from build123d import *

# Parameters (mm, degrees)
SKETCH1_R           = 6.35
BOSS_EXTRUDE1_DEPTH = 36.195
CHAMFER1_SIZE       = 4.92
CHAMFER2_SIZE       = 1.016
FILLET1_R           = 1.016
SKETCH2_R           = 10.4775
CUT_EXTRUDE1_DEPTH  = 3.175
CUT_EXTRUDE2_START  = -3.175
SKETCH3_R           = 10.4775
CUT_EXTRUDE2_DEPTH  = 3.175
SKETCH4_R           = 2.1082
CUT_EXTRUDE3_DEPTH  = 29.337
CHAMFER3_SIZE       = 1.016


with BuildPart() as part:
    # Sketch1 → Boss-Extrude1 (new body)
    with BuildSketch(Plane(origin=(0, 0, 0), x_dir=(1, 0, 0), z_dir=(0, 1, 0))):
        Polygon((-21, -13.97), (-6.985, -13.97), (-6.985, -13.208), (6.985, -13.208), (6.985, -13.97), (21, -13.97), (21, -5.194), (19.939, -5.194), (19.939, 9.011817488), (11.049, 9.011817488), (11.049, 13.97), (-11.049, 13.97), (-11.049, 9.011817488), (-19.939, 9.011817488), (-19.939, -5.194), (-21, -5.194), align=None)
        with Locations(Location((0, 1.27, 0), (0, 0, 270))):
            Circle(SKETCH1_R, mode=Mode.SUBTRACT)
    extrude(amount=BOSS_EXTRUDE1_DEPTH)

    # Chamfer1
    chamfer1_edges = [part.edges().sort_by_distance(p)[0] for p in [
        (-11.049, 18.0975, -13.97),
        (11.049, 18.0975, -13.97),
    ]]
    chamfer(chamfer1_edges, length=CHAMFER1_SIZE)

    # Chamfer2
    # the kernel refuses this chamfer: 1.016 mm, written as the material it takes off along each edge
    with BuildSketch(Plane(origin=(6.985, -2.612829916, 13.97), x_dir=(0.9996219169112968, 0, 0.027495876610587285), z_dir=(0, 1, 0))) as chamfer2_piece_1_section:
        Polygon((CHAMFER2_SIZE * 0.999621916911, CHAMFER2_SIZE * 0.0274958766106), (-CHAMFER2_SIZE * 0.0274958766106, CHAMFER2_SIZE * 0.999621916911), (0, 0), align=None)
    chamfer2_piece_1 = extrude(amount=41.420659832, mode=Mode.PRIVATE)
    chamfer2_piece_1 = split(chamfer2_piece_1, bisect_by=Plane(origin=(7.342590456, 18.0975, 13.208), z_dir=(0, 0, 1)), keep=Keep.TOP, mode=Mode.PRIVATE)
    add(chamfer2_piece_1, mode=Mode.SUBTRACT)
    with BuildSketch(Plane(origin=(-6.985, -2.612829916, 13.97), x_dir=(0.027495876610586455, 0, -0.9996219169112968), z_dir=(0, 1, 0))) as chamfer2_piece_2_section:
        Polygon((CHAMFER2_SIZE * 0.999621916911, CHAMFER2_SIZE * 0.0274958766106), (-CHAMFER2_SIZE * 0.0274958766106, CHAMFER2_SIZE * 0.999621916911), (0, 0), align=None)
    chamfer2_piece_2 = extrude(amount=41.420659832, mode=Mode.PRIVATE)
    chamfer2_piece_2 = split(chamfer2_piece_2, bisect_by=Plane(origin=(-7.342590456, 18.0975, 13.208), z_dir=(0, 0, 1)), keep=Keep.TOP, mode=Mode.PRIVATE)
    add(chamfer2_piece_2, mode=Mode.SUBTRACT)
    with BuildSketch(Plane(origin=(-21, -2.612829916, 5.194), x_dir=(0.9996219169112968, 0, -0.02749587661058551), z_dir=(0, 1, 0))) as chamfer2_piece_3:
        Polygon((CHAMFER2_SIZE * 0.999621916911, -CHAMFER2_SIZE * 0.0274958766106), (-CHAMFER2_SIZE * 0.0274958766106, -CHAMFER2_SIZE * 0.999621916911), (0, 0), align=None)
    extrude(amount=41.420659832, mode=Mode.SUBTRACT)
    with BuildSketch(Plane(origin=(21, -2.612829916, 5.194), x_dir=(-0.9996219169112968, 0, -0.027495876610584665), z_dir=(0, 1, 0))) as chamfer2_piece_4:
        Polygon((CHAMFER2_SIZE * 0.999621916911, CHAMFER2_SIZE * 0.0274958766106), (-CHAMFER2_SIZE * 0.0274958766106, CHAMFER2_SIZE * 0.999621916911), (0, 0), align=None)
    extrude(amount=41.420659832, mode=Mode.SUBTRACT)

    # Fillet1
    fillet1_edges = [part.edges().sort_by_distance(p)[0] for p in [
        (-19.939, 18.0975, -9.011817488),
        (19.939, 18.0975, -9.011817488),
        (-6.129, 18.0975, -13.97),
        (6.129, 18.0975, -13.97),
    ]]
    fillet(fillet1_edges, radius=FILLET1_R)

    # Sketch2 → Cut-Extrude1 (cut)
    with BuildSketch(Plane(origin=(0, 36.195, 0), x_dir=(1, 0, 0), z_dir=(0, 1, 0))):
        with Locations(Location((0, 1.27, 0), (0, 0, 270))):
            Circle(SKETCH2_R)
    extrude(amount=-CUT_EXTRUDE1_DEPTH, mode=Mode.SUBTRACT)

    # Sketch3 → Cut-Extrude2 (cut)
    with BuildSketch(Plane.XZ.offset(CUT_EXTRUDE2_START)):
        with Locations(Location((0, -1.27, 0), (0, 0, 90))):
            Circle(SKETCH3_R)
    extrude(amount=CUT_EXTRUDE2_DEPTH, mode=Mode.SUBTRACT)

    # Sketch4 → Cut-Extrude3 (cut)
    with BuildSketch(Plane(origin=(0, 0, -9.011817488), x_dir=(-1, 0, 0), z_dir=(0, 0, -1))):
        with Locations((-15.875, 4.7625)):
            Circle(SKETCH4_R)
        with Locations((-15.875, 31.4325)):
            Circle(SKETCH4_R)
        with Locations((15.875, 31.4325)):
            Circle(SKETCH4_R)
        with Locations((15.875, 4.7625)):
            Circle(SKETCH4_R)
    extrude(amount=-CUT_EXTRUDE3_DEPTH, mode=Mode.SUBTRACT)

    # Chamfer3
    # the kernel refuses this chamfer: 1.016 mm, written as the material it takes off along each edge
    with BuildSketch(Plane(origin=(-15.875, 4.7625, -9.011817488), x_dir=(-1, 0, 0), z_dir=(0, -1, 0))) as chamfer3_piece_1:
        Polygon((2.1082 + CHAMFER3_SIZE, 0), (2.1082, -CHAMFER3_SIZE), (2.1082, 0), align=None)
    revolve(axis=Axis((-15.875, 4.7625, -9.011817488), (0, 0, -1)), mode=Mode.SUBTRACT)
    with BuildSketch(Plane(origin=(-15.875, 31.4325, -9.011817488), x_dir=(-1, 0, 0), z_dir=(0, -1, 0))) as chamfer3_piece_2:
        Polygon((2.1082 + CHAMFER3_SIZE, 0), (2.1082, -CHAMFER3_SIZE), (2.1082, 0), align=None)
    revolve(axis=Axis((-15.875, 31.4325, -9.011817488), (0, 0, -1)), mode=Mode.SUBTRACT)
    with BuildSketch(Plane(origin=(15.875, 31.4325, -9.011817488), x_dir=(-1, 0, 0), z_dir=(0, -1, 0))) as chamfer3_piece_3:
        Polygon((2.1082 + CHAMFER3_SIZE, 0), (2.1082, -CHAMFER3_SIZE), (2.1082, 0), align=None)
    revolve(axis=Axis((15.875, 31.4325, -9.011817488), (0, 0, -1)), mode=Mode.SUBTRACT)
    with BuildSketch(Plane(origin=(15.875, 4.7625, -9.011817488), x_dir=(-1, 0, 0), z_dir=(0, -1, 0))) as chamfer3_piece_4:
        Polygon((2.1082 + CHAMFER3_SIZE, 0), (2.1082, -CHAMFER3_SIZE), (2.1082, 0), align=None)
    revolve(axis=Axis((15.875, 4.7625, -9.011817488), (0, 0, -1)), mode=Mode.SUBTRACT)


solid = part.part
Can you work these out from the model? Positions are in its coordinate system, mm. A direction names the side the tool comes from. Coordinates: 2 decimals unless noted, no trailing zeros. Loops run counter-clockwise (first coordinate to the right, second up) from the corner with the lowest first, then second, coordinate; pieces in that order, holes last. Notation, with made-up numbers: (50.5, -39.75) - (68.5, -39.75) arc R23 cw to (68.5, -25.75) - close; hole circle Ø2 at (24.25, 66.25). An arc over 180 degrees is marked (long way). Put each result on its own line as item: value. Start each with the question number.
Item 1: Suppose I cut it at A-A (z = 3.5). Please give me the cut outline in (x, y) (1 decimal), and give its area (3 significant figures).
Item 2: Suppose I cut it at C-C (x = 0). Please give me the cut outline in (y, z) (1 decimal), and give its area (3 significant figures).
Item 3: For pin 1 (6 mm diameter, centred on x = -6, z = -5, fed in from +Y); pin 2 (1 mm diameter, centred on x = 1, y = 7.5, fed in from +Z); pin 3 (2 mm diameter, centred on x = -9.5, y = 9, fed in from -Z), each with a flat end and sliding along its axis, tell me the tip position at first contact or that it passes through.
Item 4: If we mould it in two halves opening along Z, with no side actions, what happens to faces 5 (the face through (-5, 33.02, 3)), 6 (the face through (-19.939, 18, -1)), 7 (the face through (0, 18, 13.208))? For each: +Z half, -Z half, draft (parallel to the pull), parting line (faces both ways), or undercut.
Item 5: Which directions (+Z, -Z, +X, -X, +Y, -Y) give clear straight access to the entire face, cutting with the end or side of a thin tool? Please do faces 1 (the face through (19.939, 18, -1)), 2 (the face through (5, 3.175, 3)), 3 (the face through (0.461, 34.63, -11.737)), 4 (the face through (-5, 0, 9)).
Item 6: If I drill on line 1 along X through (y, z) = (30, 5.5); line 2 along X through (y, z) = (0.7, -1.27); line 3 along Y through (x, z) = (-17, -7) (3 decimals), over which ranges is the centre line in solid material (lowest first)?
Item 7: Suppose I cut it at D-D (z = -8.5). Please give me the cut outline in (x, y) (1 decimal).
Here are the results:
1. outline: (-19.9, 0) - (-9.3, 0) - (-9.3, 3.2) - (-4.2, 3.2) - (-4.2, 33) - (-9.3, 33) - (-9.3, 36.2) - (-19.9, 36.2) - close; (4.2, 3.2) - (9.3, 3.2) - (9.3, 0) - (19.9, 0) - (19.9, 36.2) - (9.3, 36.2) - (9.3, 33) - (4.2, 33) - close; hole circle Ø4.2 at (-15.9, 4.8); hole circle Ø4.2 at (-15.9, 31.4); hole circle Ø4.2 at (15.9, 4.8); hole circle Ø4.2 at (15.9, 31.4)
1. area: 1,020 mm²
2. outline: (0, -14) - (36.2, -14) - (36.2, -11.7) - (33, -11.7) - (33, -7.6) - (3.2, -7.6) - (3.2, -11.7) - (0, -11.7) - close; (0, 9.2) - (3.2, 9.2) - (3.2, 5.1) - (33, 5.1) - (33, 9.2) - (36.2, 9.2) - (36.2, 13.2) - (0, 13.2) - close
2. area: 472 mm²
3. pin 1: y = 33.02
3. pin 2: z = 13.21
3. pin 3: z = -11.6
4. face 5: undercut
4. face 6: draft
4. face 7: +Z half
5. face 1: -Z, +X, +Y, -Y
5. face 2: -Y
5. face 3: +Y
5. face 4: +Z, -Z, +X, -X, -Y
6. line 1: -20.29 to -17.42, -14.33 to 14.33, 17.42 to 20.29
6. line 2: -19.94 to -10.48, 10.48 to 19.94
6. line 3: 0 to 2.98, 6.545 to 29.65, 33.215 to 36.195
7. outline: (-19.8, 0) - (-7.6, 0) - (-7.6, 3.2) - (7.6, 3.2) - (7.6, 0) - (19.8, 0) - (19.8, 36.2) - (7.6, 36.2) - (7.6, 33) - (-7.6, 33) - (-7.6, 36.2) - (-19.8, 36.2) - close; hole circle Ø5.2 at (-15.9, 4.8); hole circle Ø5.2 at (-15.9, 31.4); hole circle Ø5.2 at (15.9, 4.8); hole circle Ø5.2 at (15.9, 31.4)
